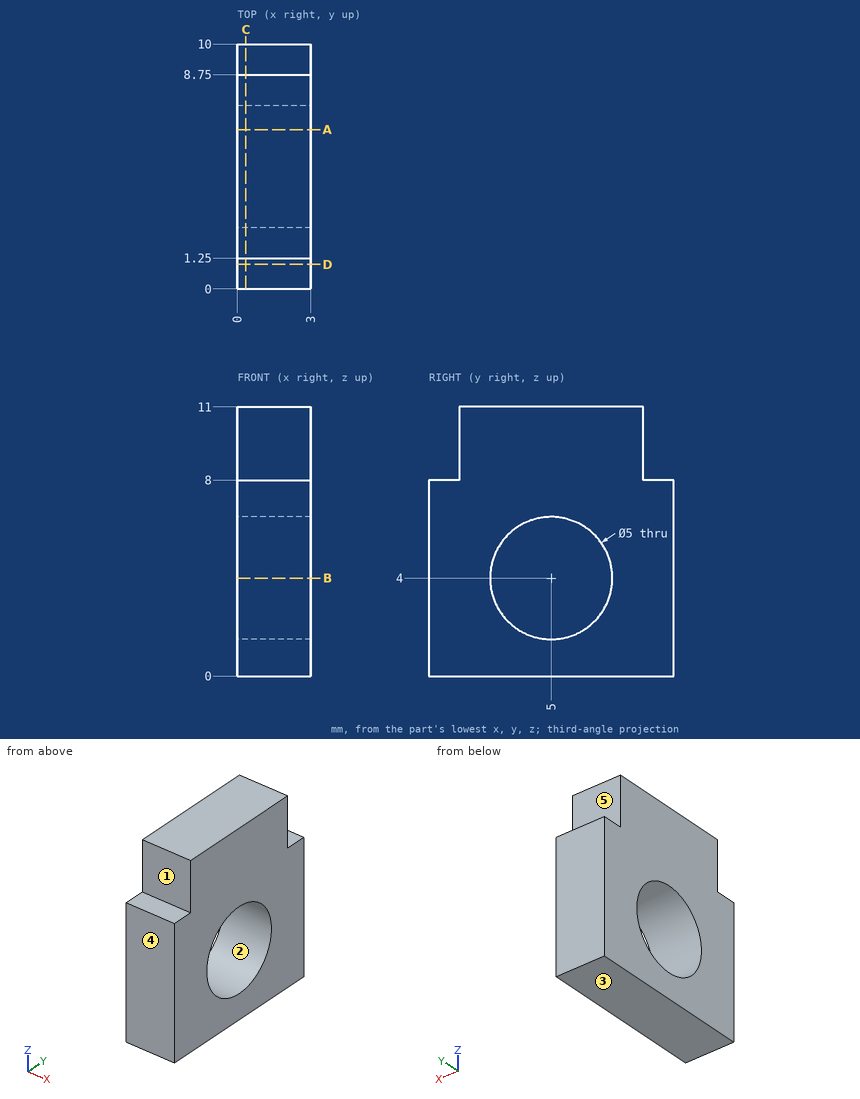
Source: three-view drawing plus pictorial views. Frame: mm from the lowest corner of the part. A direction names the side the tool comes from. Give positions to 0.01 mm unless a question says otherwise; leave off trailing zeros. Write each loop counter-clockwise with the first axis right and the second up, starting at its lowest first coordinate (ties: lowest second). Pieces come first, ordered by that corner, then holes. Notation, with made-up numbers: (74, -0.5) - (107, -0.5) arc R12 cw to (107, 7.5) - close; hole circle Ø2 at (62, 31.25). An arc over 180 degrees is marked (long way). Write item = value, one per line. Start each with the question number.
1. Section query A-A, the plane y = 6.5. Output: boundary loops of the cut face in (x, z), then the cut area to 3 significant figures.
2. Mould query, pull axis Y, two halves, no side actions, for the marked faces 1, 2 and 3. Classes: released by +Y, released by -Y, zero draft, split by the parting line, or undercut.
3. Ray query, L1, parallel to Z at x = 1.75, y = 5; L2, parallel to Y at x = 0.7, z = 4.25; L3, parallel to Y at x = 1.9, z = 5.5. Return the intervals inside material, ascending.
4. Access query for the marked faces 4 and 5. Directions: +Z, -Z, +X, -X, +Y, -Y. A direction counts if a zero-diameter tool reaches every point of the face in a straight line with its end or side. Return the directions, or none.
5. First-contact query: pin 1 Ø1 at (x, y) = (2, 0.5) entering from +Z; pin 2 Ø1.5 at (x, z) = (1, 9) entering from +Y. Flat tips, straight axial feed; report the tip coordinate or a pass-through.
6. Section query B-B, the plane z = 4. Output: boundary loops of the cut face in (x, y).
7. Section query D-D, the plane y = 1. Output: boundary loops of the cut face in (x, z).
8. Section query C-C, the plane x = 0.35. Output: boundary loops of the cut face in (y, z).
Check sheet entries:
q1.outline = (0, 0) - (3, 0) - (3, 2) - (0, 2) - close; (0, 6) - (3, 6) - (3, 11) - (0, 11) - close
q1.area = 21.0 mm2
q2.face_1 = released by -Y
q2.face_2 = undercut
q2.face_3 = zero draft
q3.L1 = 0 to 1.5, 6.5 to 11
q3.L2 = 0 to 2.51, 7.49 to 10
q3.L3 = 0 to 3, 7 to 10
q4.face_4 = +Z, -Z, +X, -X, -Y
q4.face_5 = +Z, +X, -X, +Y
q5.pin_1 = 8
q5.pin_2 = 8.75
q6.outline = (0, 0) - (3, 0) - (3, 2.5) - (0, 2.5) - close; (0, 7.5) - (3, 7.5) - (3, 10) - (0, 10) - close
q7.outline = (0, 0) - (3, 0) - (3, 8) - (0, 8) - close
q8.outline = (0, 0) - (10, 0) - (10, 8) - (8.75, 8) - (8.75, 11) - (1.25, 11) - (1.25, 8) - (0, 8) - close; hole circle Ø5 at (5, 4)
